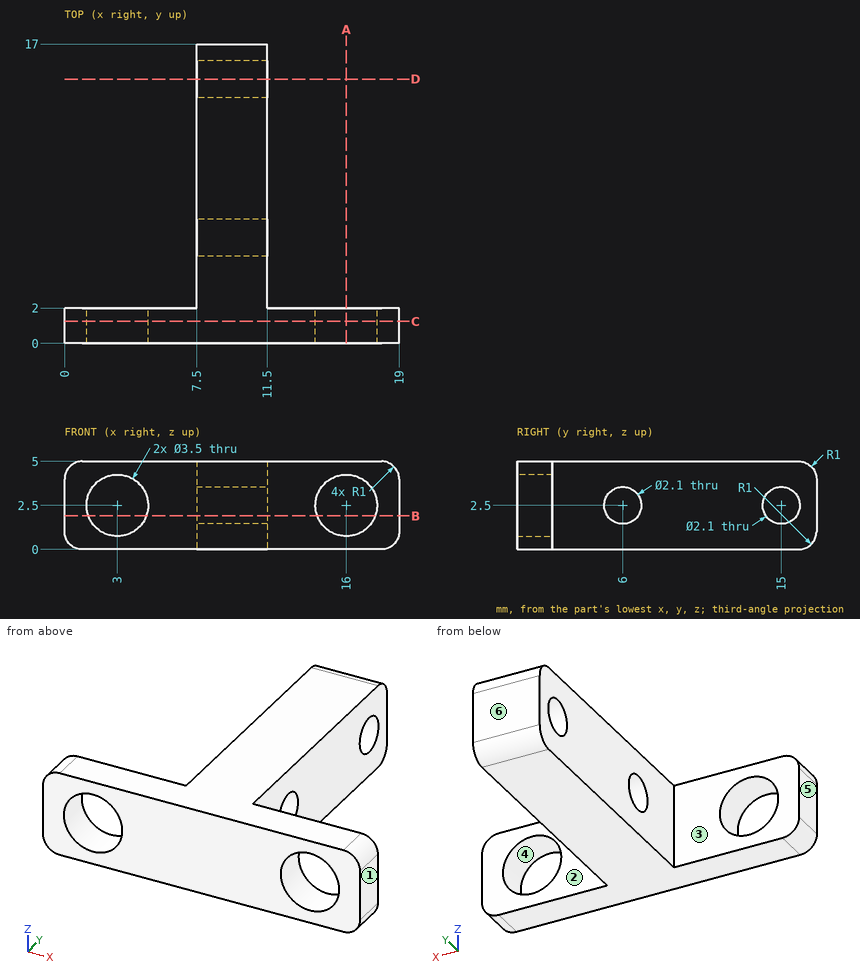
Job drawing, mm, ordinate dimensions from the low corner. One solid piece. A direction names the side the tool comes from. Give positions to 0.01 mm unless a question says otherwise; leave off trailing zeros. Loops run counter-clockwise (first coordinate to the right, second up) from the corner with the lowest first, then second, coordinate; pieces in that order, holes last. Notation, with made-up numbers: (74, 82) -> (93, 82) arc R18 ccw to (93, 94) -> close; hole circle Ø4 at (14, 22). An arc over 180 degrees is marked (long way). Use a Markdown table: item, result. Add a question column.
(1) Drop flat-ended pins along their axis: pin 1 Ø2.5 at (y, z) = (6.5, 3) entering from +X; pin 2 Ø2 at (x, z) = (5, 1.5) entering from -Y; pin 3 Ø1.5 at (x, z) = (15.5, 1.5) entering from +Y; pin 4 Ø3 at (y, z) = (7, 4.5) entering from -X. Give the stop position or say it passes through.
(2) Slice it at B-B on z = 1.9. List the corners of the cut face in (x, y).
(3) Tool access for the marked faces 1, 2 and 3: list every direction of +Z, -Z, +X, -X, +Y, -Y with a clear straight run to the whole face (end or side of a thin tool).
(4) Wall check: line 1 along X through (y, z) = (1.45, 2.5); line 2 along Y through (x, z) = (8.5, 3.35); line 3 along Y through (x, z) = (7.25, 3.65). Give the ranges that are in metal, low to high.
(5) Slice it at D-D on y = 15. List the corners of the cut face in (x, z).
(6) Slice it at C-C on y = 1.25. List the corners of the cut face in (x, z), and give its area (3 significant figures).
(7) Slice it at A-A on x = 16. List the corners of the cut face in (y, z).
(8) Mould opens along X. For the marked faces 4, 5 and 6 say: +X half, -X half, draft (parallel to the pull), parting line (faces both ways), or undercut.
Filled sheet:
| question | item | result |
|---|---|---|
| 1 | pin 1 | x = 11.5 |
| 1 | pin 2 | y = 0 |
| 1 | pin 3 | y = 2 |
| 1 | pin 4 | x = 7.5 |
| 2 | outline | (0, 0) -> (1.36, 0) -> (1.36, 2) -> (0, 2) -> close; (4.64, 0) -> (14.36, 0) -> (14.36, 2) -> (11.5, 2) -> (11.5, 5.14) -> (7.5, 5.14) -> (7.5, 2) -> (4.64, 2) -> close; (7.5, 6.86) -> (11.5, 6.86) -> (11.5, 14.14) -> (7.5, 14.14) -> close; (7.5, 15.86) -> (11.5, 15.86) -> (11.5, 17) -> (7.5, 17) -> close; (17.64, 0) -> (19, 0) -> (19, 2) -> (17.64, 2) -> close |
| 3 | face 1 | +Z, -Z, +X, +Y, -Y |
| 3 | face 2 | +Z, -Z, +X, +Y |
| 3 | face 3 | +Z, -Z, -X, +Y |
| 4 | line 1 | 0 to 1.25, 4.75 to 14.25, 17.75 to 19 |
| 4 | line 2 | 0 to 5.38, 6.62 to 14.38, 15.62 to 17 |
| 4 | line 3 | 0 to 2 |
| 5 | outline | (7.5, 0) -> (11.5, 0) -> (11.5, 1.45) -> (7.5, 1.45) -> close; (7.5, 3.55) -> (11.5, 3.55) -> (11.5, 5) -> (7.5, 5) -> close |
| 6 | outline | (0, 1) arc R1 ccw to (1, 0) -> (18, 0) arc R1 ccw to (19, 1) -> (19, 4) arc R1 ccw to (18, 5) -> (1, 5) arc R1 ccw to (0, 4) -> close; hole circle Ø3.5 at (3, 2.5); hole circle Ø3.5 at (16, 2.5) |
| 6 | area | 74.9 mm2 |
| 7 | outline | (0, 0) -> (2, 0) -> (2, 0.75) -> (0, 0.75) -> close; (0, 4.25) -> (2, 4.25) -> (2, 5) -> (0, 5) -> close |
| 8 | face 4 | undercut |
| 8 | face 5 | -X half |
| 8 | face 6 | draft |
